Verification items for the finished model (mm, model axes). Face numbers are marked on the shaded views. A direction names the side the tool comes from. Round coordinates to 2 decimals unless told otherwise and drop trailing zeros. Write each loop counter-clockwise with the first axis right and the second up, starting at its lowest first coordinate (ties: lowest second). Pieces come first, ordered by that corner, then holes. Notation, with made-up numbers: M -35.75,64 L -21.75,64 A4 ccw -21.75,69 Z; hole C 73.5,83 d11. An arc over 180 degrees is marked long. One line per item, written item: value. Start each with the question number.
Item 1: Section check D-D, the plane y = 11. Record the cut outline in (x, z).
Item 2: Gauge pin test, flat ends, axial feed: pin 1 (1 mm diameter, centred on x = 0.5, y = 3.5, fed in from -Z); pin 2 (1 mm diameter, centred on y = 9.5, z = 1, fed in from -X); pin 3 (1.5 mm diameter, centred on x = 0, y = 12.5, fed in from +Z). Record the tip position at first contact, or that the pin passes through.
Item 3: Section check B-B, the plane y = 0. Record the cut outline in (x, z), then the cut area to 3 significant figures.
Item 4: Section check A-A, the plane x = 0. Record the cut outline in (y, z), then the cut area to 3 significant figures.
Item 5: Thickness scan on probe 1 along Z at (x, y) = (5.25, 1); probe 2 along Y at (x, z) = (2.5, 0.1); probe 3 along Y at (x, z) = (1.75, 1.2). Record the ranges inside material, lowest first. Write a range as from..to.
Item 6: Section check C-C, the plane z = 0.7. Record the cut outline in (x, y).
Item 7: Tool access check on the marked faces 1 and 2. Record the directions out of +Z, -Z, +X, -X, +Y, -Y that give a thin tool (end or side, any length) a straight path to the whole face; none if there is none.
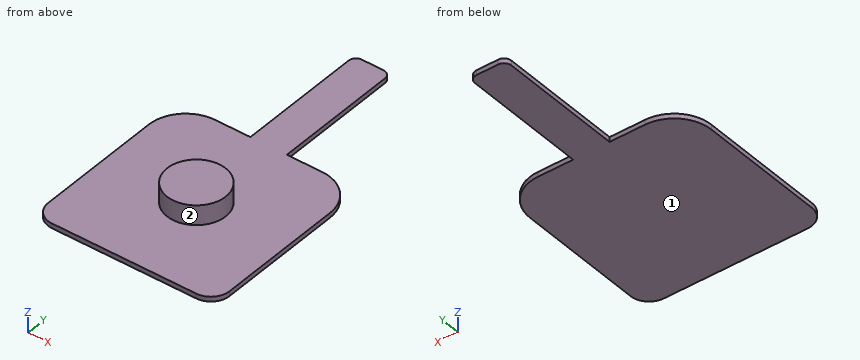
Solid Edge part; units mm, degrees
sketch "Sketch1" plane through (0, 0, 0) normal (0, 0, 1) x (1, 0, 0)
  line L0 (6.1976, 3.7084) -> (6.1976, -4.9781)
  arc A0 (6.1976, -4.9781) -> (4.9273, -6.2484) centre (4.9273, -4.9781) cw
  line L1 (4.9273, -6.2484) -> (-4.9273, -6.2484)
  arc A1 (-4.9273, -6.2484) -> (-6.1976, -4.9781) centre (-4.9273, -4.9781) cw
  line L2 (-6.1976, -4.9781) -> (-6.1976, 3.7084)
  arc A2 (-3.6576, 6.2484) -> (-6.1976, 3.7084) centre (-3.6576, 3.7084) ccw
  line L3 (-3.6576, 6.2484) -> (-1.2446, 6.2484)
  line L4 (-1.2446, 6.2484) -> (-1.2446, 14.732)
  arc A3 (-0.7366, 15.24) -> (-1.2446, 14.732) centre (-0.7366, 14.732) ccw
  line L5 (-0.7366, 15.24) -> (0.7366, 15.24)
  arc A4 (0.7366, 15.24) -> (1.2446, 14.732) centre (0.7366, 14.732) cw
  line L6 (1.2446, 14.732) -> (1.2446, 6.2484)
  line L7 (1.2446, 6.2484) -> (3.6576, 6.2484)
  arc A5 (3.6576, 6.2484) -> (6.1976, 3.7084) centre (3.6576, 3.7084) cw
extrude "Protrusion1" add sketch "Sketch1" along normal blind 0.3302
sketch "Sketch2" plane through (0, 0, 0) normal (0, 0, 1) x (1, 0, 0)
  circle A0 centre (0, 0) radius 2
extrude "ExtrudedCutout_1" add sketch "Sketch2" along normal blind 1.6764
Response values:
1. outline: M -1.24,0 L 1.24,0 L 1.24,0.33 L -1.24,0.33 Z
2. pin 1: stops at z = 0
2. pin 2: passes through
2. pin 3: stops at z = 0.33
3. outline: M -6.2,0 L 6.2,0 L 6.2,0.33 L 2,0.33 L 2,1.68 L -2,1.68 L -2,0.33 L -6.2,0.33 Z
3. area: 9.48 mm2
4. outline: M -6.25,0 L 15.24,0 L 15.24,0.33 L 2,0.33 L 2,1.68 L -2,1.68 L -2,0.33 L -6.25,0.33 Z
4. area: 12.5 mm2
5. probe 1: z = 0..0.33
5. probe 2: y = -6.25..6.25
5. probe 3: y = -0.97..0.97
6. outline: C 0,0 d4
7. face 1: -Z, +X, -X, +Y, -Y
7. face 2: +Z
